```python
from build123d import *

# Parameters (mm, degrees)
EXTRUDE1_DEPTH     = 50.8
CUT_EXTRUDE1_DEPTH = 9.525
SKETCH3_R          = 2.38125
CUT_EXTRUDE2_DEPTH = 15.875
CUT_EXTRUDE3_START = -15.875
SKETCH4_R          = 2.38125
CUT_EXTRUDE3_DEPTH = 15.875
CUT_EXTRUDE4_DEPTH = 222.795964766
EXTRUDE2_DEPTH     = 50.8


with BuildPart() as part:
    # Sketch1 → Extrude1 (new body)
    with BuildSketch(Plane.XY):
        Polygon((0, 0), (215.526146874, 0), (202.826146874, 12.7), (5.260512242, 12.7), align=None)
    extrude(amount=EXTRUDE1_DEPTH)

    # Sketch2 → Cut-Extrude1 (cut)
    with BuildSketch(Plane(origin=(0, 12.7, 0), x_dir=(-1, 0, 0), z_dir=(0, 1, 0))):
        with BuildLine():
            Line((-113.210512242, 50.8), (-62.410512242, 50.8))
            Line((-62.410512242, 50.8), (-62.410512242, 41.275))
            Line((-62.410512242, 41.275), (-24.310512242, 41.275))
            ThreePointArc((-24.310512242, 41.275), (-19.820384182, 39.415128061), (-17.960512242, 34.925))
            Line((-17.960512242, 34.925), (-17.960512242, 15.875))
            ThreePointArc((-17.960512242, 15.875), (-19.820384182, 11.384871939), (-24.310512242, 9.525))
            Line((-24.310512242, 9.525), (-106.860512242, 9.525))
            ThreePointArc((-106.860512242, 9.525), (-111.350640303, 11.384871939), (-113.210512242, 15.875))
            Line((-113.210512242, 15.875), (-113.210512242, 50.8))
        make_face()
        with BuildLine():
            Line((-132.260512242, 9.525), (-183.776146874, 9.525))
            ThreePointArc((-183.776146874, 9.525), (-188.266274935, 11.384871939), (-190.126146874, 15.875))
            Line((-190.126146874, 15.875), (-190.126146874, 34.925))
            ThreePointArc((-190.126146874, 34.925), (-188.266274935, 39.415128061), (-183.776146874, 41.275))
            Line((-183.776146874, 41.275), (-132.260512242, 41.275))
            ThreePointArc((-132.260512242, 41.275), (-127.770384182, 39.415128061), (-125.910512242, 34.925))
            Line((-125.910512242, 34.925), (-125.910512242, 15.875))
            ThreePointArc((-125.910512242, 15.875), (-127.770384182, 11.384871939), (-132.260512242, 9.525))
        make_face()
    extrude(amount=-CUT_EXTRUDE1_DEPTH, mode=Mode.SUBTRACT)

    # Sketch3 → Cut-Extrude2 (cut)
    with BuildSketch(Plane(origin=(0, 0, 0), x_dir=(-1, 0, 0), z_dir=(0, 0, -1))):
        with Locations((-120.276146874, 6.35)):
            Circle(SKETCH3_R)
    extrude(amount=-CUT_EXTRUDE2_DEPTH, mode=Mode.SUBTRACT)

    # Sketch4 → Cut-Extrude3 (cut)
    with BuildSketch(Plane.XY.offset(50.8).offset(CUT_EXTRUDE3_START)):
        with Locations(Location((120.276146874, 6.35, 0), (0, 0, 180))):
            Circle(SKETCH4_R)
    extrude(amount=CUT_EXTRUDE3_DEPTH, mode=Mode.SUBTRACT)

    # Sketch5 → Cut-Extrude4 (cut, through all)
    with BuildSketch(Plane.XY.offset(50.8)):
        with BuildLine():
            Line((0.800865302, 1.933459874), (0, 0))
            Line((0, 0), (10.521024484, 0))
            ThreePointArc((10.521024484, 0), (5.565730305, 0.488053878), (0.800865302, 1.933459874))
        make_face()
    extrude(amount=-CUT_EXTRUDE4_DEPTH, mode=Mode.SUBTRACT)

    # Sketch6 → Extrude2 (add)
    with BuildSketch(Plane.XY.offset(50.8)):
        with BuildLine():
            Line((5.660944893, 13.666729937), (5.260512242, 12.7))
            Line((5.260512242, 12.7), (10.521024484, 12.7))
            ThreePointArc((10.521024484, 12.7), (8.043377395, 12.944026939), (5.660944893, 13.666729937))
        make_face()
    extrude(amount=-EXTRUDE2_DEPTH)


solid = part.part
```
Input: part model. Units: mm. Frame: model coordinates. A direction names the side the tool comes from. Coordinates: 2 decimals unless noted, no trailing zeros. Loops run counter-clockwise (first coordinate to the right, second up) from the corner with the lowest first, then second, coordinate; pieces in that order, holes last. Notation, with made-up numbers: M 1.25,9.5 L 5.25,9.5 A34 ccw 5.25,39.5 Z; hole C 84,44 d9. An arc over 180 degrees is marked long. Use a Markdown table: item, result. Add a question column.
1) Line query: L1, parallel to Z at x = 180, y = 8 (3 decimals); L2, parallel to X at y = 4.25, z = 15; L3, parallel to X at y = 8, z = 26.5. Output: solid intervals per line, ascending. Write a range as from..to.
2) Section B-B, the plane x = 160.5. Return the cut outline in (y, z) (3 decimals).
3) Section D-D, the plane z = 25. Return the cut outline in (x, y) (3 decimals).
4) Section A-A, the plane z = 4.5. Return the cut outline in (x, y).
5) Pin query (flat end, axial travel): P1, Ø1.5, axis at y = 8.5, z = 38, coming from the -X side; P2, Ø3, axis at x = 155, y = 9, coming from the -Z side; P3, Ø12.5, axis at x = 59, z = 23, coming from the +Y side (3 decimals); P4, Ø3, axis at x = 120.28, y = 6.35, coming from the +Z side (3 decimals). Return the tip coordinate at first contact, or that it passes through.
6) Draft query along Y for faces 1 (the cylindrical face through (5.634, 0.475, 25.756)), 2 (the flat face through (120, 6, 34.925)), 3 (the cylindrical face through (118.005, 5.635, 42.751)), 4 (the cylindrical face through (19.87, 8.004, 39.464)). Return one class per face: +Y half, -Y half, draft (parallel to the pull), parting line (faces both ways), or undercut.
7) Set-up query: faces 5 (the flat face through (120, 6, 15.875)), 6 (the cylindrical face through (127.82, 8.004, 39.464)), 7 (the flat face through (113.211, 8, 33)). Return all of +Z, -Z, +X, -X, +Y, -Y with unobstructed straight access to the full face (end or side cutting, diameter ignored); none if empty.
Answer below:
| question | item | result |
|---|---|---|
| 1 | L1 | 0..9.525, 41.275..50.8 |
| 1 | L2 | 1.76..18.02, 113.15..119.15, 121.4..125.97, 190.07..211.28 |
| 1 | L3 | 3.31..17.96, 113.21..125.91, 190.13..207.53 |
| 2 | outline | M 0,0 L 12.7,0 L 12.7,9.525 L 3.175,9.525 L 3.175,41.275 L 12.7,41.275 L 12.7,50.8 L 0,50.8 Z |
| 3 | outline | M 0.801,1.933 A25.4 ccw 10.521,0 L 215.526,0 L 202.826,12.7 L 190.126,12.7 L 190.126,3.175 L 125.911,3.175 L 125.911,12.7 L 113.211,12.7 L 113.211,3.175 L 17.961,3.175 L 17.961,12.7 L 10.521,12.7 A12.7 cw 5.661,13.667 Z |
| 4 | outline | M 0.8,1.93 A25.4 ccw 10.52,0 L 215.53,0 L 202.83,12.7 L 10.52,12.7 A12.7 cw 5.66,13.67 Z; hole C 120.28,6.35 d4.76 |
| 5 | P1 | x = 3.21 |
| 5 | P2 | z = 0 |
| 5 | P3 | y = 3.175 |
| 5 | P4 | z = 34.925 |
| 6 | face 1 | -Y half |
| 6 | face 2 | undercut |
| 6 | face 3 | undercut |
| 6 | face 4 | draft |
| 7 | face 5 | -Z |
| 7 | face 6 | +Y |
| 7 | face 7 | +Z, +Y |
